Build history of the part. All positions in model axes, mm. Coordinates: 2 decimals unless noted, no trailing zeros. Order: outer loops, then holes, each group sorted by start corner. A loop starts at its lowest first (then second) coordinate and runs counter-clockwise, first axis right, second up. Notation, with made-up numbers: (3.5, 48.25) -> (58.5, 48.25) arc R18 ccw to (58.5, 59.25) -> close; hole circle Ø5 at (70, 78.5). An arc over 180 degrees is marked (long way). Write each question's results on one line, items separated by ' | '.
from build123d import *

# Parameters (mm, degrees)
SKETCH017_W     = 16
SKETCH017_H     = 15.8
PAD010_DEPTH    = 28.8
POCKET007_DEPTH = 16
PAD137_DEPTH    = 15.8
SKETCH190_W     = 16
SKETCH190_H     = 2
POCKET072_DEPTH = 30


with BuildPart() as part:
    # Sketch017 (on Face68 of Binder006) → Pad010 (new body)
    with BuildSketch(Plane.XY.offset(-28.8)):
        with Locations((-8, 127.9)):
            Rectangle(SKETCH017_W, SKETCH017_H)
    extrude(amount=PAD010_DEPTH)

    # Sketch018 (on Face3 of Pad010) → Pocket007 (cut)
    with BuildSketch(Plane.XZ.offset(-120)):
        Polygon((0, 0), (-16, -9.6), (-16, 0), align=None)
    extrude(amount=-POCKET007_DEPTH, mode=Mode.SUBTRACT)

    # Sketch141 (on Face6 of Pocket007) → Pad137 (join)
    with BuildSketch(Plane.XZ.offset(-120)):
        Polygon((0, 0), (-3.2, 0), (-16, -7.68), (-16, -10.88), (-3.2, -3.2), (0, -3.2), align=None)
    extrude(amount=-PAD137_DEPTH)

    # Sketch190 (on Face1 of Pad137) → Pocket072 (cut)
    with BuildSketch(Plane(origin=(0, 0, -28.8), x_dir=(1, 0, 0), z_dir=(0, 0, -1))):
        with Locations((-8, -121)):
            Rectangle(SKETCH190_W, SKETCH190_H)
    extrude(amount=-POCKET072_DEPTH, mode=Mode.SUBTRACT)


solid = part.part
Item 1: Slice it at C-C, the plane z = -2.75. List the corners of the cut face in (x, y), and give its area (3 significant figures).
Answer:
outline: (-7.78, 122) -> (0, 122) -> (0, 135.8) -> (-7.78, 135.8) -> close | area: 107 mm^2
Item 2: Slice it at A-A, the plane y = 123.25. List the corners of the cut face in (x, z).
Answer:
outline: (-16, -28.8) -> (0, -28.8) -> (0, 0) -> (-3.2, 0) -> (-16, -7.68) -> close
Item 3: Drill centre lines: line 1 (Z direction, x = -14.5, y = 128); line 2 (Z direction, x = -10.25, y = 135.25); line 3 (X direction, y = 125.75, z = -4.75). Where is each one in solid material? Low to high. Write a range as from..to.
Answer:
line 1: z = -28.8..-6.78 | line 2: z = -28.8..-4.23 | line 3: x = -11.12..0
Item 4: Slice it at B-B, the plane x = -12.25. List the corners of the cut face in (y, z), and give its area (3 significant figures).
Answer:
outline: (122, -28.8) -> (135.8, -28.8) -> (135.8, -5.43) -> (122, -5.43) -> close | area: 323 mm^2
Item 5: Pin check, flat tip, straight feed: pin 1 (4 mm diameter, centred on x = -9, y = 134.5, fed in from +Z). Stop position of the tip, or through.
Answer:
pin 1: stops at z = -2.28
